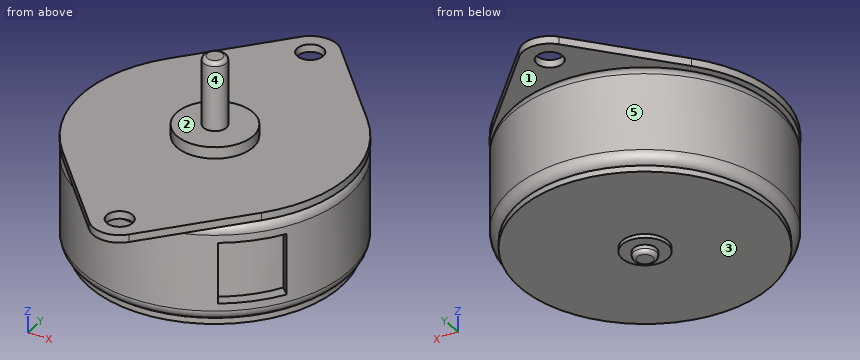
```python
from build123d import *

# Parameters (mm, degrees)
SKETCH1_R           = 1.7
BOSS_EXTRUDE1_DEPTH = 1
SKETCH2_R           = 17.5
BOSS_EXTRUDE2_DEPTH = 13
FILLET4_R           = 1.5
SKETCH3_R           = 16.5
BOSS_EXTRUDE3_DEPTH = 0.8
SKETCH4_R           = 5
BOSS_EXTRUDE4_DEPTH = 1.5
SKETCH6_R           = 1.5
BOSS_EXTRUDE5_DEPTH = 9
FILLET2_R           = 0.5
SKETCH8_R           = 3
BOSS_EXTRUDE6_DEPTH = 0.5
BOSS_EXTRUDE7_START = 1
SKETCH9_R           = 1.5
BOSS_EXTRUDE7_DEPTH = 1
FILLET3_R           = 0.5
SURFACECUT1_START   = -10.5
SURFACECUT1_DEPTH   = 8


# Read off the part's stored shape, not the designer's step: SurfaceCut1
with BuildPart() as part:
    # Sketch1 → Boss-Extrude1 (new body)
    with BuildSketch(Plane.XY):
        with BuildLine():
            Line((-13.043729869, 11.666666667), (-2.608745974, 23.333333333))
            ThreePointArc((-2.608745974, 23.333333333), (0, 24.5), (2.608745974, 23.333333333))
            Line((2.608745974, 23.333333333), (13.043729869, 11.666666667))
            ThreePointArc((13.043729869, 11.666666667), (17.5, 0), (13.043729869, -11.666666667))
            Line((13.043729869, -11.666666667), (2.608745974, -23.333333333))
            ThreePointArc((2.608745974, -23.333333333), (0, -24.5), (-2.608745974, -23.333333333))
            Line((-2.608745974, -23.333333333), (-13.043729869, -11.666666667))
            ThreePointArc((-13.043729869, -11.666666667), (-17.5, 0), (-13.043729869, 11.666666667))
        make_face()
        with Locations((0, 21)):
            Circle(SKETCH1_R, mode=Mode.SUBTRACT)
        with Locations((0, -21)):
            Circle(SKETCH1_R, mode=Mode.SUBTRACT)
    extrude(amount=BOSS_EXTRUDE1_DEPTH)


with BuildPart() as body_2:
    # Sketch2 → Boss-Extrude2 (new body)
    with BuildSketch(Plane(origin=(0, 0, 0), x_dir=(-1, 0, 0), z_dir=(0, 0, -1))):
        with Locations(Location((0, 0, 0), (0, 0, 180))):
            Circle(SKETCH2_R)
    extrude(amount=BOSS_EXTRUDE2_DEPTH)

    # Fillet4
    fillet4_edges = [body_2.edges().sort_by_distance(p)[0] for p in [
        (-17.5, 0, 0),
        (-17.5, 0, -13),
    ]]
    fillet(fillet4_edges, radius=FILLET4_R)


with BuildPart() as part_1:
    add(part.part)

    # Combine1: union body 2
    add(body_2.part)

    # Sketch3 → Boss-Extrude3 (add)
    with BuildSketch(Plane(origin=(0, 0, -13), x_dir=(-1, 0, 0), z_dir=(0, 0, -1))):
        Circle(SKETCH3_R)
    extrude(amount=BOSS_EXTRUDE3_DEPTH)

    # Sketch4 → Boss-Extrude4 (add)
    with BuildSketch(Plane.XY.offset(1)):
        Circle(SKETCH4_R)
    extrude(amount=BOSS_EXTRUDE4_DEPTH)

    # Sketch6 → Boss-Extrude5 (add)
    with BuildSketch(Plane.XY.offset(2.5)):
        Circle(SKETCH6_R)
    extrude(amount=BOSS_EXTRUDE5_DEPTH)

    # Fillet2
    fillet2_edges = [part_1.edges().sort_by_distance(p)[0] for p in [
        (-1.5, 0, 11.5),
    ]]
    fillet(fillet2_edges, radius=FILLET2_R)

    # Sketch8 → Boss-Extrude6 (add)
    with BuildSketch(Plane(origin=(0, 0, -13.8), x_dir=(-1, 0, 0), z_dir=(0, 0, -1))):
        Circle(SKETCH8_R)
    extrude(amount=BOSS_EXTRUDE6_DEPTH)

    # Sketch9 → Boss-Extrude7 (add)
    with BuildSketch(Plane(origin=(0, 0, -14.3), x_dir=(-1, 0, 0), z_dir=(0, 0, -1)).offset(BOSS_EXTRUDE7_START)):
        with Locations(Location((0, 0, 0), (0, 0, 180))):
            Circle(SKETCH9_R)
    extrude(amount=-BOSS_EXTRUDE7_DEPTH)

    # Fillet3
    fillet3_edges = [part_1.edges().sort_by_distance(p)[0] for p in [
        (-1.5, 0, -15.3),
    ]]
    fillet(fillet3_edges, radius=FILLET3_R)

    # SurfaceCut1 outline → SurfaceCut1 (cut)
    with BuildSketch(Plane.XY.offset(SURFACECUT1_START)):
        with BuildLine():
            Line((8.126024025, -13.782878275), (9.218356678, -14.875210928))
            ThreePointArc((9.218356678, -14.875210928), (12.374368671, -12.374368671), (14.875210928, -9.218356678))
            Line((14.875210928, -9.218356678), (13.782878275, -8.126024025))
            ThreePointArc((13.782878275, -8.126024025), (11.313708499, -11.313708499), (8.126024025, -13.782878275))
        make_face()
    extrude(amount=SURFACECUT1_DEPTH, mode=Mode.SUBTRACT)


solid = part_1.part
```
For this review, take the finished solid that the model builds, in its own axes (mm). Face numbers are marked on the shaded views. A direction names the side the tool comes from. Give positions to 0.01 mm unless a question says otherwise; leave off trailing zeros. Write each loop counter-clockwise with the first axis right and the second up, starting at its lowest first coordinate (ties: lowest second). Pieces come first, ordered by that corner, then holes. Notation, with made-up numbers: M -40,-1.75 L 11,-1.75 A26 ccw 11,30.25 Z; hole C 18.5,30 d11. An arc over 180 degrees is marked long. One line per item, written item: value.
1) For line 1 (Y direction, x = 0, z = 0.35); line 2 (Z direction, x = 13, y = -5.5); line 3 (Z direction, x = 2, y = -19.5), list the stretches that pass through material, from the lowest coordinate up. Write a range as from..to.
Results are:
line 1: y = -24.5..-22.7, -19.3..19.3, 22.7..24.5
line 2: z = -13.8..1
line 3: z = 0..1
2) Take a section at B-B, the plane x = 0. Count the separate pieces of the cut face and the enclosed holes in it, then the cut area to 3 significant figures.
Results are:
separate pieces: 3
enclosed holes: 0
area: 569 mm²
3) Take a section at A-A, the plane y = -21. Write out the cut boundary in (x, z), then the cut area to 3 significant figures.
Results are:
outline: M -4.7,0 L -1.7,0 L -1.7,1 L -4.7,1 Z; M 1.7,0 L 4.7,0 L 4.7,1 L 1.7,1 Z
area: 5.99 mm²
4) For P1, Ø4, axis at y = -18, z = -3, coming from the +X side; P2, Ø8, axis at x = -11.5, z = -4, coming from the +Y side; P3, Ø1, axis at x = -10, y = -16, coming from the +Z side; P4, Ø4, axis at x = -3.5, y = -2, coming from the -Z side, all flat-tipped, find the tip position at first contact; note any pin that passes through.
Results are:
P1: stops at x = 7.09
P2: stops at y = 15.81
P3: passes through
P4: stops at z = -14.3
5) The part is to be moulded in two halves that separate along Z. For the marked faces 1, 2 and 3, say which applies: +Z half, -Z half, draft (parallel to the pull), parting line (faces both ways), or undercut.
Results are:
face 1: undercut
face 2: +Z half
face 3: -Z half
6) For the marked faces 4 and 5, list the 3-axis set-ups (+Z, -Z, +X, -X, +Y, -Y) from which the entire face can be reached by the end or side of a thin tool; tool diameter is ignored.
Results are:
face 4: +Z
face 5: -Z
7) Take a section at C-C, the plane z = -5.75. Write out the cut boundary in (x, y).
Results are:
outline: M 8.13,-13.78 A16 ccw 13.78,-8.13 L 14.88,-9.22 A17.5 ccw long 9.22,-14.88 Z
